```python
from build123d import *

# Parameters (mm, degrees)
ESBO_O1_W                                           = 30
ESBO_O1_H                                           = 30
RESSALTO_EXTRUS_O1_DEPTH                            = 50
ESBO_O2_W                                           = 25
ESBO_O2_H                                           = 5
CORTE_EXTRUS_O1_DEPTH                               = 31
CORTE_EXTRUS_O2_START                               = -5
ESBO_O3_W                                           = 25
ESBO_O3_H                                           = 25
CORTE_EXTRUS_O2_DEPTH                               = 26
FURO_COM_FOLGA_DE_M41_D                             = 4.5
FURO_COM_FOLGA_DE_M41_ON_FACE_2_D                   = 4.5
ESBO_O5_W                                           = 30
ESBO_O5_H                                           = 10
RESSALTO_EXTRUS_O2_DEPTH                            = 12
REBAIXO_PARA_PARAFUSO_COM_CABE_A_PANELA_D           = 3.4
REBAIXO_PARA_PARAFUSO_COM_CABE_A_PANELA_CBORE_D     = 7
REBAIXO_PARA_PARAFUSO_COM_CABE_A_PANELA_CBORE_DEPTH = 2.4


with BuildPart() as part:
    # Esboço1 → Ressalto-extrusão1 (new body)
    with BuildSketch(Plane.XY):
        with Locations((-15, 15)):
            Rectangle(ESBO_O1_W, ESBO_O1_H)
    extrude(amount=RESSALTO_EXTRUS_O1_DEPTH)

    # Esboço2 → Corte-extrusão1 (cut, through all)
    with BuildSketch(Plane(origin=(0, 30, 0), x_dir=(1, 0, 0), z_dir=(0, 1, 0))):
        with Locations((-17.5, -12.5)):
            Rectangle(ESBO_O2_W, ESBO_O2_H)
    extrude(amount=-CORTE_EXTRUS_O1_DEPTH, mode=Mode.SUBTRACT)

    # Esboço3 → Corte-extrusão2 (cut, through all)
    with BuildSketch(Plane(origin=(0, 30, 0), x_dir=(1, 0, 0), z_dir=(0, 1, 0)).offset(CORTE_EXTRUS_O2_START)):
        with Locations((-17.5, -37.5)):
            Rectangle(ESBO_O3_W, ESBO_O3_H)
    extrude(amount=-CORTE_EXTRUS_O2_DEPTH, mode=Mode.SUBTRACT)

    # Furo com folga de M41 (through all)
    with Locations(Plane(origin=(-5, 15, 35), x_dir=(0, 0, -1), z_dir=(-1, 0, 0))):
        with Locations((0, 0)):
            Hole(FURO_COM_FOLGA_DE_M41_D / 2)

    # Furo com folga de M41 on face 2 (through all)
    with Locations(Plane(origin=(-15, 25, 35), x_dir=(0, 0, -1), z_dir=(0, -1, 0))):
        with Locations((0, 0)):
            Hole(FURO_COM_FOLGA_DE_M41_ON_FACE_2_D / 2)

    # Esboço5 → Ressalto-extrusão2 (add)
    with BuildSketch(Plane(origin=(0, 30, 0), x_dir=(1, 0, 0), z_dir=(0, 1, 0))):
        with Locations((-15, -5)):
            Rectangle(ESBO_O5_W, ESBO_O5_H)
    extrude(amount=RESSALTO_EXTRUS_O2_DEPTH)

    # Rebaixo para parafuso com cabeça panela de M31 (through all)
    with Locations(Plane(origin=(0, 0, 0), x_dir=(-1, 0, 0), z_dir=(0, 0, -1))):
        with Locations((15, 36)):
            CounterBoreHole(REBAIXO_PARA_PARAFUSO_COM_CABE_A_PANELA_D / 2, REBAIXO_PARA_PARAFUSO_COM_CABE_A_PANELA_CBORE_D / 2, REBAIXO_PARA_PARAFUSO_COM_CABE_A_PANELA_CBORE_DEPTH)


solid = part.part
```
Could you check a few things on this model? Use its own coordinates, in mm. A direction names the side the tool comes from. Round coordinates to 2 decimals unless told otherwise and drop trailing zeros. Loops run counter-clockwise (first coordinate to the right, second up) from the corner with the lowest first, then second, coordinate; pieces in that order, holes last. Notation, with made-up numbers: M -34,-28 L -3,-28 A37 ccw -3,10 Z; hole C -5.5,-0.75 d4. An arc over 180 degrees is marked long. Put each result on its own line as item: value.
Q1. Imagine slicing it at B-B (x = -3). Write out the boundary of the cut face in (y, z), then the cut area to 3 significant figures.
Check result:
outline: M 0,0 L 42,0 L 42,10 L 30,10 L 30,50 L 0,50 Z; hole C 15,35 d4.5
area: 1,600 mm2
Q2. Imagine slicing it at C-C (y = 28.5). Write out the boundary of the cut face in (x, z).
Check result:
outline: M -30,0 L 0,0 L 0,50 L -30,50 L -30,15 L -5,15 L -5,10 L -30,10 Z; hole C -15,35 d4.5
Q3. On a 3-axis mill with a long thin cutter (end or side, diameter ignored), from which of +Z, -Z, +X, -X, +Y, -Y can I reach the whole of each face in a straight line? I mean faces 5 (the face through (-15, 30, 30)), 6 (the face through (-5, 15, 13)), 7 (the face through (-14.54, 39.47, 1.18)). Say none if no direction works.
Check result:
face 5: +Z, +X, -X, +Y
face 6: -X, +Y, -Y
face 7: -Z
Q4. Thinking about a two-plate mould opening in Z: for faces 1 (the face through (-15.86, 27.53, 37.08)), 2 (the face through (-2.47, 15.86, 37.08)), 3 (the face through (-18, 13, 25)), 4 (the face through (-15, 42, 5)), which applies, released by +Z, released by -Z, zero draft, split by the parting line, or undercut?
Check result:
face 1: undercut
face 2: undercut
face 3: released by +Z
face 4: zero draft
Q5. For pin 1 (8 mm diameter, centred on x = -10.5, y = 12.5, fed in from +Z); pin 2 (4 mm diameter, centred on x = -15, y = 36, fed in from +Z); pin 3 (2.5 mm diameter, centred on y = 9.5, z = 11.5, fed in from -X), each with a flat end and sliding along its axis, tell me the tip position at first contact or that it passes through.
Check result:
pin 1: z = 25
pin 2: z = 10
pin 3: x = -5
Q6. Imagine slicing it at D-D (z = 35). Write out the boundary of the cut face in (x, y).
Check result:
outline: M -30,25 L -17.25,25 L -17.25,30 L -30,30 Z; M -12.75,25 L -5,25 L -5,17.25 L 0,17.25 L 0,30 L -12.75,30 Z; M -5,0 L 0,0 L 0,12.75 L -5,12.75 Z
Q7. I need wall thicknesses on probe 1 along Z at (x, y) = (-9.25, 14); probe 2 along Y at (x, z) = (-15, 8.5); probe 3 along Z at (x, y) = (-22.25, 28). Which ranges of each line are inside material? Lowest first, please.
Check result:
probe 1: 0 to 10, 15 to 25
probe 2: 0 to 34.3, 37.7 to 42
probe 3: 0 to 10, 15 to 50
Q8. Imagine slicing it at A-A (y = 15). Write out the boundary of the cut face in (x, z), then the cut area to 4 significant figures.
Check result:
outline: M -30,0 L 0,0 L 0,32.75 L -5,32.75 L -5,25 L -30,25 L -30,15 L -5,15 L -5,10 L -30,10 Z; M -5,37.25 L 0,37.25 L 0,50 L -5,50 Z
area: 727.5 mm2
